The listing builds one solid part. Answer for the finished solid, in the listing's coordinates (mm). A direction names the side the tool comes from. Give positions to 0.01 mm unless a question says otherwise; leave off trailing zeros. Order: outer loops, then holes, each group sorted by start corner. A loop starts at its lowest first (then second) coordinate and runs counter-clockwise, first axis right, second up.
```python
from build123d import *

# Parameters (mm, degrees)
CYLINDER830_R                                           = 2.5
CYLINDER830_DEPTH                                       = 38
CYLINDER832_R                                           = 2.3
CYLINDER832_DEPTH                                       = 2
CYLINDER831_R                                           = 2
CYLINDER831_DEPTH                                       = 0.5
CYLINDER833_R                                           = 1.75
CYLINDER833_DEPTH                                       = 6
CYLINDER834_R                                           = 1
CYLINDER834_DEPTH                                       = 11
CYLINDER828_R                                           = 2
CYLINDER828_DEPTH                                       = 3.5
FUSION088026007031024007008004081022014_PLACEMENT_ANGLE = 180


with BuildPart() as cylinder:
    # Cylinder830 → Cylinder830 (new body)
    with BuildSketch(Plane.XZ.offset(-86.5)):
        Circle(CYLINDER830_R)
    extrude(amount=CYLINDER830_DEPTH)


with BuildPart() as cylinder832:
    # Cylinder832 → Cylinder832 (new body)
    with BuildSketch(Plane.XZ.offset(-48)):
        Circle(CYLINDER832_R)
    extrude(amount=CYLINDER832_DEPTH)


with BuildPart() as cylinder831:
    # Cylinder831 → Cylinder831 (new body)
    with BuildSketch(Plane.XZ.offset(-48.5)):
        Circle(CYLINDER831_R)
    extrude(amount=CYLINDER831_DEPTH)


with BuildPart() as sphere:
    # Sphere → Sphere (revolve)
    with BuildSketch(Plane.XZ.offset(-39.5)):
        with BuildLine():
            ThreePointArc((0, -3), (3, 0), (0, 3))
            Line((0, 3), (0, -3))
        make_face()
    revolve(axis=Axis((0, 39.5, 0), (0, 0, 1)))


with BuildPart() as cylinder833:
    # Cylinder833 → Cylinder833 (new body)
    with BuildSketch(Plane.XZ.offset(-46)):
        Circle(CYLINDER833_R)
    extrude(amount=CYLINDER833_DEPTH)


with BuildPart() as cylinder834:
    # Cylinder834 → Cylinder834 (new body)
    with BuildSketch(Plane(origin=(0, 39.5, -5.5), x_dir=(0, 1, 0), z_dir=(0, 0, 1))):
        Circle(CYLINDER834_R)
    extrude(amount=CYLINDER834_DEPTH)


with BuildPart() as axle_shaft_left:
    # Cylinder828 → Cylinder828 (new body)
    with BuildSketch(Plane.XZ.offset(-90)):
        Circle(CYLINDER828_R)
    extrude(amount=CYLINDER828_DEPTH)

    # Fusion088026007031024007008004081022014: union Cylinder, Cylinder832, Cylinder831, Sphere, Cylinder833, Cylinder834
    add(cylinder.part)
    add(cylinder832.part)
    add(cylinder831.part)
    add(sphere.part)
    add(cylinder833.part)
    add(cylinder834.part)


with BuildPart() as axle_shaft_left_1:
    # Fusion088026007031024007008004081022014 placement: moved
    add(axle_shaft_left.part.moved(Location((75, 93, 46))).rotate(Axis((75, 93, 46), (0, 0, 1)), FUSION088026007031024007008004081022014_PLACEMENT_ANGLE))


solid = axle_shaft_left_1.part
```
1) Find section D-D (y = 9.5). Write down the section's boundary in (x, z).
Geometry says:
outline: circle Ø5 at (75, 46)
2) A tool of negligible diameter and unlimited length cuts with its end or side. For faces 1 (the flat face through (75, 54, 40.5)), 2 (the cylindrical face through (77, 25.2, 44.5)), 3 (the cylindrical face through (74.024, 53.717, 41.817)), 4 (the flat face through (75, 54, 51.5)), 5 (the cylindrical face through (74.19, 49, 44.45)), from which of +Z, -Z, +X, -X, +Y, -Y can it reach the whole face along a straight path? Write none if from no direction.
Geometry says:
face 1: -Z, +X, -X, +Y, -Y
face 2: -Y
face 3: -Z
face 4: +Z, +X, -X, +Y, -Y
face 5: none
3) Find section C-C (z = 50.75). Write down the section's boundary in (x, y), then the cut area to 3 significant figures.
Geometry says:
outline: circle Ø2 at (75, 53.5)
area: 3.14 mm2
4) Straight lines are drawn through the part: probe 1 along Y at (x, z) = (74.6, 44); probe 2 along Y at (x, z) = (74.2, 48); probe 3 along Z at (x, y) = (74.9, 46.5). For each, find the intervals that lie inside material, in ascending order.
Geometry says:
probe 1: y = 6.5 to 44.5, 45 to 47, 51.3 to 55.7
probe 2: y = 6.5 to 44.5, 45 to 47, 51.41 to 55.59
probe 3: z = 43.7 to 48.3
5) Find section A-A (z = 46). Write down the section's boundary in (x, y), then the cut area to 3 significant figures.
Geometry says:
outline: (72.5, 6.5) - (73, 6.5) - (73, 3) - (77, 3) - (77, 6.5) - (77.5, 6.5) - (77.5, 44.5) - (77, 44.5) - (77, 45) - (77.3, 45) - (77.3, 47) - (76.75, 47) - (76.75, 51.06) arc R3 ccw (long way) to (73.25, 51.06) - (73.25, 47) - (72.7, 47) - (72.7, 45) - (73, 45) - (73, 44.5) - (72.5, 44.5) - close
area: 256 mm2
6) Find section B-B (y = 53.5). Write down the section's boundary in (x, z), then the cut area to 3 significant figures.
Geometry says:
outline: (74, 40.5) - (76, 40.5) - (76, 43.17) arc R3 ccw to (76, 48.83) - (76, 51.5) - (74, 51.5) - (74, 48.83) arc R3 ccw to (74, 43.17) - close
area: 38.5 mm2
7) For a pull along Y with two mould halves and no side action, classify faces 6 (the cylindrical face through (74.024, 53.717, 50.146)), 7 (the cylindrical face through (73.153, 4.726, 45.234)), 8 (the cylindrical face through (73.153, 44.747, 45.234)) as +Y half, -Y half, draft (parallel to the pull), parting line (faces both ways), or undercut.
Geometry says:
face 6: parting line
face 7: draft
face 8: undercut
8) Given P1, Ø6, axis at y = 30, z = 47.5, coming from the +X side; P2, Ø1.5, axis at x = 76, z = 45, coming from the +Y side; P3, Ø2, axis at x = 75.5, z = 49.5, coming from the +Y side, each flat-ended and moving along its own axis, determine where each tip first touches the part or whether it passes through.
Geometry says:
P1: stops at x = 77.5
P2: stops at y = 56.43
P3: stops at y = 55.1
